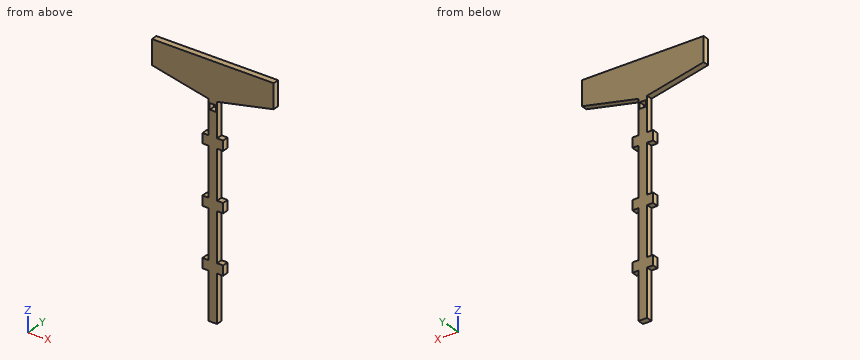
```python
from build123d import *

# Parameters (mm, degrees)
SKETCH1_W           = 6.35
SKETCH1_H           = 6.35
BOSS_EXTRUDE2_DEPTH = 6.35


with BuildPart() as part:
    # Sketch1 → Boss-Extrude2 (new body)
    with BuildSketch(Plane(origin=(0, 0, 0), x_dir=(1, 0, 0), z_dir=(0, 1, 0))):
        Polygon((0, 0), (127, 0), (127, 25.4), (67.945, 38.1), (67.945, 73.566782), (74.295, 73.566782), (74.295, 83.698651246), (67.945, 83.698651246), (67.945, 134.288657), (74.295, 134.288657), (74.295, 144.420526246), (67.945, 144.420526246), (67.945, 195.010544446), (74.295, 195.010544446), (74.295, 205.142413692), (67.945, 205.142413692), (67.945, 254.126831852), (59.055, 254.126831852), (59.055, 205.142413692), (52.705, 205.142413692), (52.705, 195.010544446), (59.055, 195.010544446), (59.055, 144.420526246), (52.705, 144.420526246), (52.705, 134.288657), (59.055, 134.288657), (59.055, 83.698651246), (52.705, 83.698651246), (52.705, 73.566782), (59.055, 73.566782), (59.055, 38.1), (0, 25.4), align=None)
        with Locations((63.5, 45.085)):
            Rectangle(SKETCH1_W, SKETCH1_H, mode=Mode.SUBTRACT)
    extrude(amount=BOSS_EXTRUDE2_DEPTH)


solid = part.part
```
Work out the finished part from the listing and answer in its coordinate system (mm). Give positions to 0.01 mm unless a question says otherwise; leave off trailing zeros. Order: outer loops, then holes, each group sorted by start corner. A loop starts at its lowest first (then second) coordinate and runs counter-clockwise, first axis right, second up.
1. Section A-A, the plane x = 64 is taken. Determine the outline of the cut face in (y, z), and give its area (3 significant figures).
Result sheet:
outline: (0, -254.13) - (6.35, -254.13) - (6.35, -48.26) - (0, -48.26) - close; (0, -41.91) - (6.35, -41.91) - (6.35, 0) - (0, 0) - close
area: 1,570 mm2
2. Each of these flat-tipped pins is pushed along its axis until it touches: P1, Ø1.9, axis at x = 55.5, y = 4.5, coming from the -Z side; P2, Ø1.9, axis at y = 2, z = -139.5, coming from the -X side (3 decimals); P3, Ø1.9, axis at y = 4, z = -182.5, coming from the -X side (3 decimals). Where does it stop, or does it pass through?
Result sheet:
P1: stops at z = -205.14
P2: stops at x = 52.705
P3: stops at x = 59.055
3. Section C-C, the plane x = 10 is taken. Determine the outline of the cut face in (y, z), and give its area (3 significant figures).
Result sheet:
outline: (0, -27.55) - (6.35, -27.55) - (6.35, 0) - (0, 0) - close
area: 175 mm2
4. Section B-B, the plane z = -237 is taken. Determine the outline of the cut face in (x, y) (3 decimals).
Result sheet:
outline: (59.055, 0) - (67.945, 0) - (67.945, 6.35) - (59.055, 6.35) - close
5. Straight lines are drawn through the part: L1, parallel to Z at x = 62, y = 3.5; L2, parallel to Z at x = 73.5, y = 2; L3, parallel to X at y = 4, z = -171 (3 decimals). For each, find the intervals that lie inside material, in ascending order.
Result sheet:
L1: z = -254.13 to -48.26, -41.91 to 0
L2: z = -205.14 to -195.01, -144.42 to -134.29, -83.7 to -73.57, -36.91 to 0
L3: x = 59.055 to 67.945
